Source: CAD feature listing. Evaluate the final solid. Frame: model axes, mm. A direction names the side the tool comes from. Give positions to 0.01 mm unless a question says otherwise; leave off trailing zeros. Order: outer loops, then holes, each group sorted by start corner. A loop starts at its lowest first (then second) coordinate and runs counter-clockwise, first axis right, second up. Notation, with made-up numbers: (86.5, 19) -> (120.5, 19) arc R19 cw to (120.5, 38) -> close; hole circle Ø8 at (89.5, 72). An arc over 180 degrees is marked (long way). Use one line per item in the form item = value. Start each with the question number.
from build123d import *

# Parameters (mm, degrees)
PAD_DEPTH          = 3.65
SKETCH002_R        = 2.55
PAD002_DEPTH       = 3
SKETCH006_W        = 72
SKETCH006_H        = 38
POCKET001_DEPTH    = 1.65
SKETCH003_R        = 1.55
PAD003_DEPTH       = 1.65
CHAMFER_1_SIZE2    = 0.2
CHAMFER_1_SIZE     = 2.5
CHAMFER_2_SIZE2    = 0.2
CHAMFER_2_SIZE     = 2.5
CHAMFER001_1_SIZE2 = 0.2
CHAMFER001_1_SIZE  = 1.55
CHAMFER001_2_SIZE2 = 0.2
CHAMFER001_2_SIZE  = 1.55
POCKET_DEPTH       = 6.651


with BuildPart() as part:
    # Sketch001 → Pad (new body)
    with BuildSketch(Plane.XY):
        with BuildLine():
            Line((-51, 73.85), (-51, 0))
            ThreePointArc((-51, 0), (-49.535534, -3.535534), (-46, -5))
            Line((-46, -5), (46, -5))
            ThreePointArc((46, -5), (49.535534, -3.535534), (51, 0))
            Line((51, 0), (51, 73.85))
            ThreePointArc((51, 73.85), (49.535534, 77.385534), (46, 78.85))
            Line((46, 78.85), (-46, 78.85))
            ThreePointArc((-46, 78.85), (-49.535534, 77.385534), (-51, 73.85))
        make_face()
    extrude(amount=PAD_DEPTH)

    # Sketch002 → Pad002 (join)
    with BuildSketch(Plane.XY.offset(3.65)):
        with Locations((-15, 0)):
            Circle(SKETCH002_R)
        with Locations((15, 0)):
            Circle(SKETCH002_R)
    extrude(amount=PAD002_DEPTH)

    # Sketch006 → Pocket001 (cut)
    with BuildSketch(Plane.XY.offset(3.65)):
        with Locations((0, 45)):
            Rectangle(SKETCH006_W, SKETCH006_H)
    extrude(amount=-POCKET001_DEPTH, mode=Mode.SUBTRACT)

    # Sketch003 → Pad003 (join)
    with BuildSketch(Plane.XY.offset(2)):
        with Locations((-15, 30.2)):
            Circle(SKETCH003_R)
        with Locations((15, 30.2)):
            Circle(SKETCH003_R)
    extrude(amount=PAD003_DEPTH)

    # Chamfer 1
    chamfer_1_edges = [part.edges().sort_by_distance(p)[0] for p in [
        (-17.55, 0, 6.65),
    ]]
    chamfer_1_side = part.faces().sort_by_distance((-17.55, 0, 5.15))[0]
    chamfer(chamfer_1_edges, length=CHAMFER_1_SIZE, length2=CHAMFER_1_SIZE2, reference=chamfer_1_side)

    # Chamfer 2
    chamfer_2_edges = [part.edges().sort_by_distance(p)[0] for p in [
        (12.45, 0, 6.65),
    ]]
    chamfer_2_side = part.faces().sort_by_distance((12.45, 0, 5.15))[0]
    chamfer(chamfer_2_edges, length=CHAMFER_2_SIZE, length2=CHAMFER_2_SIZE2, reference=chamfer_2_side)

    # Chamfer001 1
    chamfer001_1_edges = [part.edges().sort_by_distance(p)[0] for p in [
        (-16.55, 30.2, 3.65),
    ]]
    chamfer001_1_side = part.faces().sort_by_distance((-16.55, 30.2, 2.825))[0]
    chamfer(chamfer001_1_edges, length=CHAMFER001_1_SIZE, length2=CHAMFER001_1_SIZE2, reference=chamfer001_1_side)

    # Chamfer001 2
    chamfer001_2_edges = [part.edges().sort_by_distance(p)[0] for p in [
        (13.45, 30.2, 3.65),
    ]]
    chamfer001_2_side = part.faces().sort_by_distance((13.45, 30.2, 2.825))[0]
    chamfer(chamfer001_2_edges, length=CHAMFER001_2_SIZE, length2=CHAMFER001_2_SIZE2, reference=chamfer001_2_side)

    # Sketch005 → Pocket (cut, through all)
    with BuildSketch(Plane.XY):
        with BuildLine():
            Line((-26, 53.1), (-26, 35.5))
            ThreePointArc((-26, 35.5), (-25.414214, 34.085786), (-24, 33.5))
            Line((-24, 33.5), (24, 33.5))
            ThreePointArc((24, 33.5), (25.414214, 34.085786), (26, 35.5))
            Line((26, 35.5), (26, 53.1))
            ThreePointArc((26, 53.1), (25.414214, 54.514214), (24, 55.1))
            Line((24, 55.1), (-24, 55.1))
            ThreePointArc((-24, 55.1), (-25.414214, 54.514214), (-26, 53.1))
        make_face()
    extrude(amount=POCKET_DEPTH, mode=Mode.SUBTRACT)


solid = part.part
1) Cut plane D-D, the plane x = 15. Return the cut outline in (y, z).
2) Cut plane C-C, the plane y = 30.2. Return the cut outline in (x, z), plus the area to 3 significant figures.
3) Cut plane B-B, the plane y = 40. Return the cut outline in (x, z), plus the area to 4 significant figures.
4) Pin query (flat end, axial travel): pin 1 (1.4 mm diameter, centred on x = 15.5, y = 30.5, fed in from +Z); pin 2 (19 mm diameter, centred on x = -16, y = 41.5, fed in from +Z). Return the tip coordinate at first contact, or that it passes through.
5) Draft query along Y for faces 4 (the face through (49.57, 77.35, 1.8)), 5 (the face through (0, 55.1, 1)), 6 (the face through (12.452, 0.112, 3.896)), 7 (the face through (-1, 28, 0)). Return one class per face: +Y half, -Y half, draft (parallel to the pull), parting line (faces both ways), or undercut.
6) Reachability of faces 1 (the face through (-1, -5, 2)), 2 (the face through (-25.43, 34.1, 0.99)), 3 (the face through (-1, 58, 2)) from +Z, -Z, +X, -X, +Y, -Y: full face, straight path, thin tool, end or side. Return the list, or none.
7) Material intervals for probe 1 along Y at (x, z) = (5, 2.25); probe 2 along X at (y, z) = (49.5, 2.75); probe 3 along Y at (x, z) = (-19, 0.5), sorted ascending.
8) Cut plane A-A, the plane x = -6. Return the cut outline in (y, z).
Output values:
q1.outline = (-5, 0) -> (33.5, 0) -> (33.5, 2) -> (31.75, 2) -> (31.75, 2.1) -> (31.55, 3.65) -> (28.85, 3.65) -> (28.65, 2.1) -> (28.65, 2) -> (26, 2) -> (26, 3.65) -> (2.55, 3.65) -> (2.55, 4.15) -> (2.35, 6.65) -> (-2.35, 6.65) -> (-2.55, 4.15) -> (-2.55, 3.65) -> (-5, 3.65) -> close; (55.1, 0) -> (78.85, 0) -> (78.85, 3.65) -> (64, 3.65) -> (64, 2) -> (55.1, 2) -> close
q2.outline = (-51, 0) -> (51, 0) -> (51, 3.65) -> (36, 3.65) -> (36, 2) -> (16.55, 2) -> (16.55, 2.1) -> (16.35, 3.65) -> (13.65, 3.65) -> (13.45, 2.1) -> (13.45, 2) -> (-13.45, 2) -> (-13.45, 2.1) -> (-13.65, 3.65) -> (-16.35, 3.65) -> (-16.55, 2.1) -> (-16.55, 2) -> (-36, 2) -> (-36, 3.65) -> (-51, 3.65) -> close
q2.area = 263 mm^2
q3.outline = (-51, 0) -> (-26, 0) -> (-26, 2) -> (-36, 2) -> (-36, 3.65) -> (-51, 3.65) -> close; (26, 0) -> (51, 0) -> (51, 3.65) -> (36, 3.65) -> (36, 2) -> (26, 2) -> close
q3.area = 149.5 mm^2
q4.pin_1 = 3.65
q4.pin_2 = 2
q5.face_4 = +Y half
q5.face_5 = undercut
q5.face_6 = parting line
q5.face_7 = draft
q6.face_1 = +Z, -Z, +X, -X, -Y
q6.face_2 = +Z, -Z
q6.face_3 = +Z
q7.probe_1 = -5 to 26, 64 to 78.85
q7.probe_2 = -51 to -36, 36 to 51
q7.probe_3 = -5 to 33.5, 55.1 to 78.85
q8.outline = (-5, 0) -> (33.5, 0) -> (33.5, 2) -> (26, 2) -> (26, 3.65) -> (-5, 3.65) -> close; (55.1, 0) -> (78.85, 0) -> (78.85, 3.65) -> (64, 3.65) -> (64, 2) -> (55.1, 2) -> close
